Model file for the job. Use its own axes, mm. Face numbers are marked on the shaded views. A direction names the side the tool comes from. Coordinates: 2 decimals unless noted, no trailing zeros. Loops run counter-clockwise (first coordinate to the right, second up) from the corner with the lowest first, then second, coordinate; pieces in that order, holes last.
from build123d import *

# Parameters (mm, degrees)
SKETCH1_W           = 43.18
SKETCH1_H           = 17.78
BOSS_EXTRUDE1_DEPTH = 12.7
CUT_EXTRUDE1_DEPTH  = 7.62
CUT_EXTRUDE2_DEPTH  = 18.78
BOSS_EXTRUDE2_DEPTH = 10.16
CUT_EXTRUDE3_DEPTH  = 7.62


with BuildPart() as part:
    # Sketch1 → Boss-Extrude1 (new body)
    with BuildSketch(Plane.XY):
        with Locations((21.59, 8.89)):
            Rectangle(SKETCH1_W, SKETCH1_H)
    extrude(amount=-BOSS_EXTRUDE1_DEPTH)

    # Sketch3 → Cut-Extrude1 (cut)
    with BuildSketch(Plane(origin=(0, 17.78, 0), x_dir=(1, 0, 0), z_dir=(0, 1, 0))):
        Polygon((43.18, 12.7), (36.83, 6.35), (43.18, 0), align=None)
    extrude(amount=-CUT_EXTRUDE1_DEPTH, mode=Mode.SUBTRACT)

    # Sketch4 → Cut-Extrude2 (cut, through all)
    with BuildSketch(Plane(origin=(0, 17.78, 0), x_dir=(1, 0, 0), z_dir=(0, 1, 0))):
        with BuildLine():
            Line((32.381000008, 4.599999944), (24.260999992, 4.599999944))
            ThreePointArc((24.260999992, 4.599999944), (22.510999936, 6.35), (24.260999992, 8.100000056))
            Line((24.260999992, 8.100000056), (32.381000008, 8.100000056))
            ThreePointArc((32.381000008, 8.100000056), (34.131000064, 6.35), (32.381000008, 4.599999944))
        make_face()
        with BuildLine():
            Line((15.68099988, 4.599999944), (7.560999864, 4.599999944))
            ThreePointArc((7.560999864, 4.599999944), (5.810999808, 6.35), (7.560999864, 8.100000056))
            Line((7.560999864, 8.100000056), (15.68099988, 8.100000056))
            ThreePointArc((15.68099988, 8.100000056), (17.430999936, 6.35), (15.68099988, 4.599999944))
        make_face()
    extrude(amount=-CUT_EXTRUDE2_DEPTH, mode=Mode.SUBTRACT)

    # Sketch5 → Boss-Extrude2 (add)
    with BuildSketch(Plane(origin=(0, 10.16, 0), x_dir=(1, 0, 0), z_dir=(0, 1, 0))):
        Polygon((43.18, 12.7), (49.53, 6.35), (43.18, 0), align=None)
    extrude(amount=-BOSS_EXTRUDE2_DEPTH)

    # Sketch6 → Cut-Extrude3 (cut)
    with BuildSketch(Plane(origin=(0, 17.78, 0), x_dir=(1, 0, 0), z_dir=(0, 1, 0))):
        with BuildLine():
            Line((41.91, 12.7), (43.18, 12.7))
            Line((43.18, 12.7), (42.281974388, 11.801974388))
            ThreePointArc((42.281974388, 11.801974388), (42.257767431, 12.317998762), (41.91, 12.7))
        make_face()
        with BuildLine():
            Line((41.91, 0), (43.18, 0))
            Line((43.18, 0), (42.281974388, 0.898025612))
            ThreePointArc((42.281974388, 0.898025612), (42.257767431, 0.382001238), (41.91, 0))
        make_face()
    extrude(amount=-CUT_EXTRUDE3_DEPTH, mode=Mode.SUBTRACT)


solid = part.part
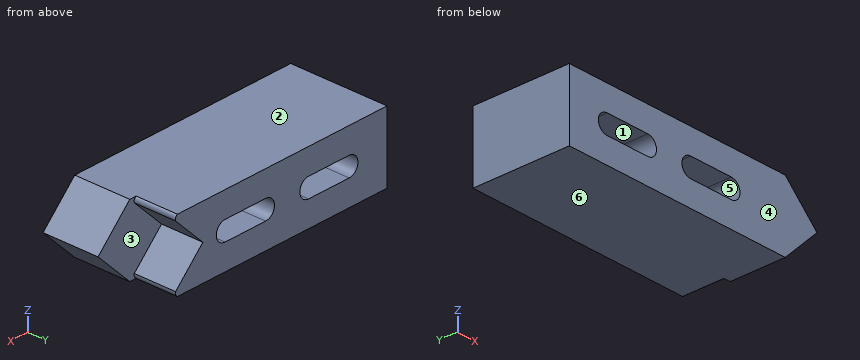
Q1. Flat gauge pins, fed straight in: P1, Ø5, axis at y = 15.5, z = -2.5, coming from the +X side; P2, Ø1.5, axis at y = 14, z = -4.5, coming from the +X side. Where does each tip first touch, or does it go through?
Answers:
P1: stops at x = 42.32
P2: stops at x = 39.43
Q2. Slice it at B-B (x = 11.5). List the corners of the cut face in (y, z), and give its area (3 significant figures).
Answers:
outline: (0, -12.7) - (17.78, -12.7) - (17.78, -8.1) - (0, -8.1) - close; (0, -4.6) - (17.78, -4.6) - (17.78, 0) - (0, 0) - close
area: 164 mm2
Q3. Which spindle directions (+Z, -Z, +X, -X, +Y, -Y) get a long thin tool onto all of the face, cutting with end or side? Do the marked faces 1, 2 and 3. Say none if no direction does.
Answers:
face 1: +Y, -Y
face 2: +Z, +X, -X, +Y, -Y
face 3: +X, +Y
Q4. Slice it at A-A (y = 3.25). List the corners of the cut face in (x, z).
Answers:
outline: (0, -12.7) - (43.18, -12.7) - (49.53, -6.35) - (43.18, 0) - (0, 0) - close; hole (7.56, -8.1) - (15.68, -8.1) arc R1.75 ccw to (15.68, -4.6) - (7.56, -4.6) arc R1.75 ccw to start; hole (24.26, -8.1) - (32.38, -8.1) arc R1.75 ccw to (32.38, -4.6) - (24.26, -4.6) arc R1.75 ccw to start
Q5. Slice it at C-C (z = -7). List the corners of the cut face in (x, y), and give its area (3 significant figures).
Answers:
outline: (0, 0) - (5.94, 0) - (5.94, 17.78) - (0, 17.78) - close; (17.31, 0) - (22.64, 0) - (22.64, 17.78) - (17.31, 17.78) - close; (34.01, 0) - (48.88, 0) - (48.88, 10.16) - (37.48, 10.16) - (37.48, 17.78) - (34.01, 17.78) - close
area: 378 mm2
Q6. Slice it at D-D (x = 33.5). List the corners of the cut face in (y, z), and give its area (3 significant figures).
Answers:
outline: (0, -12.7) - (17.78, -12.7) - (17.78, -7.7) - (0, -7.7) - close; (0, -5) - (17.78, -5) - (17.78, 0) - (0, 0) - close
area: 178 mm2
Q7. Drill centre lines: line 1 (Z direction, x = 12, y = 8.75); line 2 (X direction, y = 6.5, z = -6.5); line 3 (Y direction, x = 43.5, z = -3.5). Where is each one in solid material? Low to high.
Answers:
line 1: z = -12.7 to -8.1, -4.6 to 0
line 2: x = 0 to 5.82, 17.42 to 22.52, 34.12 to 49.38
line 3: y = 0 to 10.16
Q8. Mould opens along Z. For the marked faces 4, 5 and 6 say: +Z half, -Z half, draft (parallel to the pull), parting line (faces both ways), or undercut.
Answers:
face 4: draft
face 5: undercut
face 6: -Z half
